```python
from build123d import *

# Parameters (mm, degrees)
F0_W      = 203.2
F0_H      = 101.6
F1_DEPTH  = 76.2
F3_DEPTH  = 25.4
F2_W      = 50.8
F2_H      = 50.8
F4_DEPTH  = 76.2
F5_W      = 25.4
F5_H      = 50.8
F6_DEPTH  = 203.2
F7_DEPTH  = 25.4
F9_DEPTH  = 76.2
F11_DEPTH = 76.2


with BuildPart() as f1:
    # F0 (on Front) → F1 (new body)
    with BuildSketch(Plane.XZ):
        with Locations((27.0239350557, -1.4781945765)):
            Rectangle(F0_W, F0_H)
    extrude(amount=F1_DEPTH)

    # F3 (add): a face of the model
    f3_faces = [f1.faces().sort_by_distance(p)[0] for p in [
        (27.0239350557, 0, -1.4781945765),
    ]]
    extrude(f3_faces, amount=F3_DEPTH)

    # F2 (on face) → F4 (cut)
    with BuildSketch(Plane.XZ.offset(76.2)):
        with Locations((103.2239350557, -26.8781945765)):
            Rectangle(F2_W, F2_H)
        with Locations((-49.1760649443, -26.8781945765)):
            Rectangle(F2_W, F2_H)
    extrude(amount=-F4_DEPTH, mode=Mode.SUBTRACT)

    # F5 (on face) → F6 (cut)
    with BuildSketch(Plane.YZ.offset(128.6239350557)):
        with Locations((-63.5, 23.9218054235)):
            Rectangle(F5_W, F5_H)
    extrude(amount=-F6_DEPTH, mode=Mode.SUBTRACT)

    # F7 (add): a face of the model
    f7_faces = [f1.faces().sort_by_distance(p)[0] for p in [
        (27.0239350557, -76.2, -26.8781945765),
    ]]
    extrude(f7_faces, amount=F7_DEPTH)

    # F8 (on face) → F9 (cut)
    with BuildSketch(Plane.XZ.offset(50.8)):
        with BuildLine():
            Line((128.6239350557, 49.3218054235), (103.2239350557, 49.3218054235))
            ThreePointArc((103.2239350557, 49.3218054235), (121.1844472979, 41.8823176656), (128.6239350557, 23.9218054235))
            Line((128.6239350557, 23.9218054235), (128.6239350557, 49.3218054235))
        make_face()
        with BuildLine():
            Line((-49.1760649443, 49.3218054235), (-74.5760649443, 49.3218054235))
            Line((-74.5760649443, 49.3218054235), (-74.5760649443, 23.9218054235))
            ThreePointArc((-74.5760649443, 23.9218054235), (-67.1365771864, 41.8823176656), (-49.1760649443, 49.3218054235))
        make_face()
    extrude(amount=-F9_DEPTH, mode=Mode.SUBTRACT)

    # F10 (on face) → F11 (cut)
    with BuildSketch(Plane.XZ.offset(50.8)):
        with BuildLine():
            ThreePointArc((-36.4760649443, 23.9218054235), (-40.1958088232, 32.9020615446), (-49.1760649443, 36.6218054235))
            ThreePointArc((-49.1760649443, 36.6218054235), (-58.1563210653, 14.9415493024), (-36.4760649443, 23.9218054235))
        make_face()
        with BuildLine():
            ThreePointArc((115.9239350557, 23.9218054235), (112.2041911768, 32.9020615446), (103.2239350557, 36.6218054235))
            ThreePointArc((103.2239350557, 36.6218054235), (94.2436789347, 14.9415493024), (115.9239350557, 23.9218054235))
        make_face()
    extrude(amount=-F11_DEPTH, mode=Mode.SUBTRACT)


solid = f1.part
```
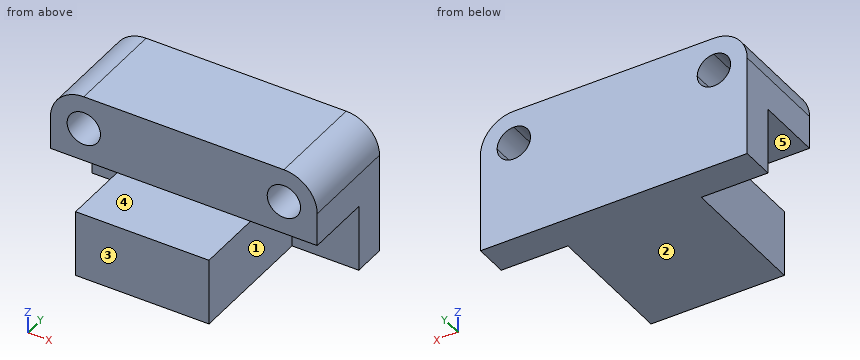
Part model, mm, in its own coordinate system. Face numbers are marked on the shaded views. A direction names the side the tool comes from. Round coordinates to 2 decimals unless told otherwise and drop trailing zeros. Order: outer loops, then holes, each group sorted by start corner. A loop starts at its lowest first (then second) coordinate and runs counter-clockwise, first axis right, second up. Notation, with made-up numbers: M 20,-12.75 L 52,-12.75 A17 ccw 52,15.25 Z; hole C -9,18.25 d11. An arc over 180 degrees is marked long. Answer in a Markdown table with one row per item. Add a question column.
Q1. Cut at A-A on y = -15.5. Give the cut face in (x, z).
Q2. Wall check: L1, parallel to Z at x = 31, y = -83; L2, parallel to Y at x = -52.5, z = -39; L3, parallel to Y at x = 118, z = 7. Give the ranges that are in metal, low to high. Write a range as from..to.
Q3. Pin check, flat tips, straight feed: pin 1 (2 mm diameter, centred on y = -64.5, z = -25.5, fed in from -X); pin 2 (15 mm diameter, centred on x = 49, z = 13, fed in from -Y); pin 3 (3 mm diameter, centred on y = 3.5, z = 39, fed in from +X). Stop position of each tip, or through.
Q4. 3-axis set-ups, long thin cutter, end or side, ignore diameter. For the marked faces 1, 2, 3, 4 and 5: which of +Z, -Z, +X, -X, +Y, -Y reach the whole face in a straight line?
Q5. Cut at D-D on z = -13.5. Give the cut face in (x, y), and give its area (3 significant figures).
Q6. Cut at B-B on x = -33.5. Give the cut face in (y, z), and give its area (3 significant figures).
Q7. Cut at C-C on z = 27. Give the cut face in (x, y).
Established:
| question | item | result |
|---|---|---|
| 1 | outline | M -74.58,-1.48 L -23.78,-1.48 L -23.78,-52.28 L 77.82,-52.28 L 77.82,-1.48 L 128.62,-1.48 L 128.62,23.92 A25.4 ccw 103.22,49.32 L -49.18,49.32 A25.4 ccw -74.58,23.92 Z; hole C -49.18,23.92 d25.4; hole C 103.22,23.92 d25.4 |
| 2 | L1 | z = -52.28..-1.48 |
| 2 | L2 | y = 0..25.4 |
| 2 | L3 | y = -50.8..25.4 |
| 3 | pin 1 | stops at x = -23.78 |
| 3 | pin 2 | stops at y = -50.8 |
| 3 | pin 3 | stops at x = 124.69 |
| 4 | face 1 | -Z, +X, -Y |
| 4 | face 2 | -Z, +X, -X, +Y, -Y |
| 4 | face 3 | +Z, -Z, +X, -X, -Y |
| 4 | face 4 | +Z, +X, -X, -Y |
| 4 | face 5 | -Z, -X, -Y |
| 5 | outline | M -74.58,0 L -23.78,0 L -23.78,-101.6 L 77.82,-101.6 L 77.82,0 L 128.62,0 L 128.62,25.4 L -74.58,25.4 Z |
| 5 | area | 15,500 mm2 |
| 6 | outline | M -50.8,-1.48 L 0,-1.48 L 0,-52.28 L 25.4,-52.28 L 25.4,49.32 L -50.8,49.32 Z |
| 6 | area | 5,160 mm2 |
| 7 | outline | M -74.39,-50.8 L -61.5,-50.8 L -61.5,25.4 L -74.39,25.4 Z; M -36.85,-50.8 L 90.9,-50.8 L 90.9,25.4 L -36.85,25.4 Z; M 115.55,-50.8 L 128.44,-50.8 L 128.44,25.4 L 115.55,25.4 Z |
